```python
from build123d import *

# Parameters (mm, degrees)
SKETCH_2_R          = 5
CUT_EXTRUDE_1_DEPTH = 60


with BuildPart() as part:
    # Эскиз1 → Повернуть1 (revolve)
    with BuildSketch(Plane.XY, mode=Mode.PRIVATE) as revolve_1_sk:
        Polygon((8, 1), (6, 1), (6, 2), (8.75, 2), (9.5, 2.75), (9.5, 4), (9, 4), (9, 4.75), (10, 4.75), (10, 10.75), (9, 11.25), (9, 15.25), (8.5, 15.75), (6, 15.75), (6, 26.75), (8.5, 26.75), (9, 27.25), (9, 31.25), (10, 31.75), (10, 37.75), (9, 37.75), (9, 38.5), (9.5, 38.5), (9.5, 39.75), (8.75, 40.5), (6, 40.5), (6, 41.5), (8, 41.5), (8, 42.5), (0, 42.5), (0, 0), (8, 0), align=None)
    revolve(revolve_1_sk.sketch.rotate(Axis((0, 136.374036199, 0), (0, -1, 0)), 90), axis=Axis((0, 136.374036199, 0), (0, -1, 0)))

    # Эскиз2 → Вырез-Вытянуть1 (cut)
    with BuildSketch(Plane(origin=(0, 42.5, 0), x_dir=(1, 0, 0), z_dir=(0, 1, 0))):
        with Locations(Location((0, 0, 0), (0, 0, 270))):
            Circle(SKETCH_2_R)
    extrude(amount=-CUT_EXTRUDE_1_DEPTH, mode=Mode.SUBTRACT)


solid = part.part
```
Here's how the part is built. I have some questions about the finished solid (model axes, mm). A direction names the side the tool comes from. Round coordinates to 2 decimals unless told otherwise and drop trailing zeros. Write each loop counter-clockwise with the first axis right and the second up, starting at its lowest first coordinate (ties: lowest second). Pieces come first, ordered by that corner, then holes.
Q1. Will these pins go through, and if not, where does the flat tip stop? P1, Ø12, axis at y = 13, z = -6, coming from the -X side; P2, Ø4, axis at x = 4, y = 6, coming from the +Z side; P3, Ø1.5, axis at x = -5, y = 14, coming from the +Z side; P4, Ø5, axis at x = 0.5, z = 0.5, coming from the -Y side.
Q2. If we section it at A-A on y = 33: Write out the boundary of the cut face in (x, z).
Q3. If we section it at B-B on x = -7.25: Give the number of separate pieces and of enclosed holes in the cut face, plus the area to 3 significant figures.
Q4. Please list where these lines run through material, in increasing order: probe 1 along Y at (x, z) = (2.5, 7.5); probe 2 along X at (y, z) = (19.5, 0); probe 3 along Y at (x, z) = (5.5, -7.25).
Q5. Which directions (+Z, -Z, +X, -X, +Y, -Y) give clear straight access to the entire face, cutting with the end or side of a thin tool? Please do faces 1 (the flat face through (5.2, 42.5, -0.1)), 2 (the cylindrical face through (7.81, 42.01, -1.73)), 3 (the cylindrical face through (0, 8, -10)), 4 (the flat face through (-6, 1, -2)), 5 (the cylindrical face through (7.81, 0.51, -1.73)).
Q6. If we section it at C-C on y = 16.5: Write out the boundary of the cut face in (x, z).
Answer below:
1. P1: stops at x = -9.99
1. P2: stops at z = 9.8
1. P3: stops at z = 7.93
1. P4: passes through
2. outline: circle Ø20 at (0, 0); hole circle Ø10 at (0, 0)
3. separate pieces: 4
3. enclosed holes: 0
3. area: 349 mm2
4. probe 1: y = 0 to 1, 2 to 15.75, 26.75 to 40.5, 41.5 to 42.5
4. probe 2: x = -6 to -5, 5 to 6
4. probe 3: y = 2.35 to 4, 4.75 to 11.2, 31.3 to 37.75, 38.5 to 40.15
5. face 1: +Z, -Z, +X, -X, +Y
5. face 2: +Y
5. face 3: +Y, -Y
5. face 4: none
5. face 5: -Y
6. outline: circle Ø12 at (0, 0); hole circle Ø10 at (0, 0)
